```python
from build123d import *

# Parameters (mm, degrees)
BOSS_EXTRUDE1_DEPTH                = 12
SKETCH2_R                          = 6
BOSS_EXTRUDE2_DEPTH                = 3
F_6_0_6_DIAMETER_HOLE2_D           = 6
F_6_0_6_DIAMETER_HOLE2_CSINK_D     = 6.05
F_6_0_6_DIAMETER_HOLE2_CSINK_ANGLE = 90
SKETCH7_R                          = 14
SKETCH7_R_2                        = 9
BOSS_EXTRUDE4_DEPTH                = 17.5
BOSS_EXTRUDE6_DEPTH                = 5
SKETCH9_R                          = 9
CUT_EXTRUDE1_DEPTH                 = 30
BOSS_EXTRUDE7_REACH                = 69.941
SKETCH10_W                         = 30
SKETCH10_H                         = 8
FILLET1_R                          = 10


with BuildPart() as part:
    # Sketch1 → Boss-Extrude1 (new body)
    with BuildSketch(Plane(origin=(0, 0, 0), x_dir=(1, 0, 0), z_dir=(0, 1, 0))):
        with BuildLine():
            Line((-34, 30), (34, 30))
            ThreePointArc((34, 30), (38.242640687, 28.242640687), (40, 24))
            Line((40, 24), (40, -24))
            ThreePointArc((40, -24), (38.242640687, -28.242640687), (34, -30))
            Line((34, -30), (-34, -30))
            ThreePointArc((-34, -30), (-38.242640687, -28.242640687), (-40, -24))
            Line((-40, -24), (-40, 24))
            ThreePointArc((-40, 24), (-38.242640687, 28.242640687), (-34, 30))
        make_face()
    extrude(amount=BOSS_EXTRUDE1_DEPTH)

    # Sketch2 → Boss-Extrude2 (add)
    with BuildSketch(Plane(origin=(0, 12, 0), x_dir=(1, 0, 0), z_dir=(0, 1, 0))):
        with Locations(Location((-34, 24, 0), (0, 0, 90))):
            Circle(SKETCH2_R)
        with Locations(Location((-34, -24, 0), (0, 0, 270))):
            Circle(SKETCH2_R)
        with Locations(Location((34, 24, 0), (0, 0, 90))):
            Circle(SKETCH2_R)
        with Locations(Location((34, -24, 0), (0, 0, 270))):
            Circle(SKETCH2_R)
    extrude(amount=BOSS_EXTRUDE2_DEPTH)

    # Ø6.0 (6) Diameter Hole2 (through all)
    with Locations(Plane(origin=(0, 15, 0), x_dir=(1, 0, 0), z_dir=(0, 1, 0))):
        with Locations((-34, 24), (34, 24), (34, -24), (-34, -24)):
            CounterSinkHole(F_6_0_6_DIAMETER_HOLE2_D / 2, F_6_0_6_DIAMETER_HOLE2_CSINK_D / 2, counter_sink_angle=F_6_0_6_DIAMETER_HOLE2_CSINK_ANGLE)


with BuildPart() as body_2:
    # Sketch7 → Boss-Extrude4 (new, symmetric)
    with BuildSketch(Plane(origin=(0, 0, 0), x_dir=(0, 0, -1), z_dir=(1, 0, 0))):
        with Locations((0, 40)):
            Circle(SKETCH7_R)
        with Locations((0, 40)):
            Circle(SKETCH7_R_2, mode=Mode.SUBTRACT)
    extrude(amount=BOSS_EXTRUDE4_DEPTH, both=True)

    # Sketch8 → Boss-Extrude6 (add, symmetric)
    with BuildSketch(Plane(origin=(0, 0, 0), x_dir=(0, 0, -1), z_dir=(1, 0, 0))):
        with BuildLine():
            Line((-18, 40), (-18, 58))
            Line((-18, 58), (18, 58))
            Line((18, 58), (18, 40))
            ThreePointArc((18, 40), (0, 22), (-18, 40))
        make_face()
    extrude(amount=BOSS_EXTRUDE6_DEPTH, both=True)

    # Sketch9 → Cut-Extrude1 (cut, symmetric)
    with BuildSketch(Plane(origin=(5, 0, 0), x_dir=(0, 0, -1), z_dir=(1, 0, 0))):
        with Locations((0, 40)):
            Circle(SKETCH9_R)
    extrude(amount=CUT_EXTRUDE1_DEPTH, both=True, mode=Mode.SUBTRACT)

    # Sketch10 → Boss-Extrude7 (add, up to next)
    with BuildSketch(Plane(origin=(0, 12, 0), x_dir=(1, 0, 0), z_dir=(0, 1, 0)), mode=Mode.PRIVATE) as boss_extrude7_sk1:
        Rectangle(SKETCH10_W, SKETCH10_H)
    boss_extrude7_tool1 = extrude(boss_extrude7_sk1.sketch, amount=BOSS_EXTRUDE7_REACH, mode=Mode.PRIVATE) - body_2.part

    add(part.part)  # Boss-Extrude7 merges part
    add(boss_extrude7_tool1.solids().sort_by_distance((0, 12, 0))[0])

    # Fillet1
    fillet1_edges = [body_2.edges().sort_by_distance(p)[0] for p in [
        (0, 58, 18),
        (0, 58, -18),
    ]]
    fillet(fillet1_edges, radius=FILLET1_R)


solid = body_2.part
```
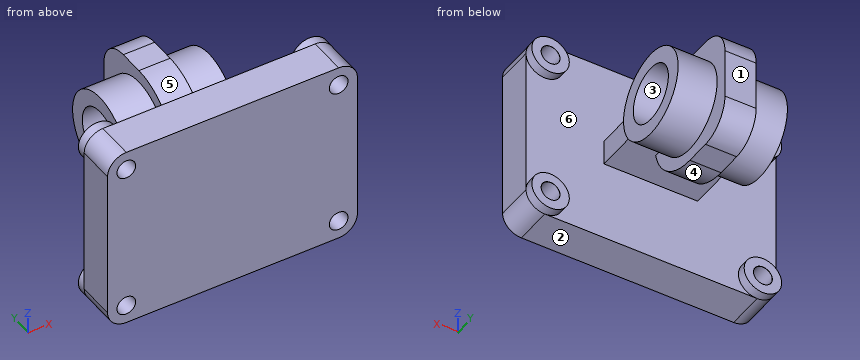
Check sheet for the modelled part. Datum: model origin and axes. Units: mm. Face numbers are marked on the shaded views. A direction names the side the tool comes from. Coordinates: 2 decimals unless noted, no trailing zeros. Order: outer loops, then holes, each group sorted by start corner. A loop starts at its lowest first (then second) coordinate and runs counter-clockwise, first axis right, second up. Notation, with made-up numbers: M 68,38.5 L 83,38.5 A9 cw 83,46.5 Z; hole C 35.25,64 d9. An arc over 180 degrees is marked long. Write each question's results on one line, items separated by ' | '. Start each with the question number.
1. Cross-section at B-B on x = 14. Record the cut outline in (y, z), and give its area (3 significant figures).
2. Access from +Z, -Z, +X, -X, +Y, -Y to the whole of each face (thin tool, end or side, straight path). Record for the marked faces 4, 5 and 6.
3. Cross-section at A-A on z = 0. Record the cut outline in (x, y).
4. Cross-section at D-D on y = 32.5. Record the cut outline in (x, z), and give its area (3 significant figures).
5. Mould release check, pull along Y, two halves, no side actions. Record for the marked faces 1, 2 and 3: +Y half, -Y half, draft (parallel to the pull), parting line (faces both ways), or undercut.
6. Cross-section at C-C on y = 9. Record the cut outline in (x, z).
7. Go/stop test with flat-tipped pins: P1, Ø18, axis at y = 32, z = -4.5, coming from the +X side; P2, Ø3.5, axis at x = -34, z = -24, coming from the +Y side; P3, Ø6, axis at x = 33.5, z = 22, coming from the +Y side; P4, Ø3, axis at x = 21.5, z = -9.5, coming from the +Y side. Record where each tip stops, or that it passes through.
8. Material ranges on probe 1 along Z at (x, y) = (34, 10); probe 2 along X at (y, z) = (4.75, -24); probe 3 along Y at (x, z) = (3, 0), recorded low to high.
Checks:
1) outline: M 0,-30 L 12,-30 L 12,-4 L 26.58,-4 A14 ccw long 26.58,4 L 12,4 L 12,30 L 0,30 Z; hole C 40,0 d18 | area: 1,190 mm²
2) face 4: -Z, +X, -X | face 5: +Z, +X, -X | face 6: none
3) outline: M -40,0 L 40,0 L 40,12 L 15,12 L 15,26 L 17.5,26 L 17.5,31 L -17.5,31 L -17.5,26 L -15,26 L -15,12 L -40,12 Z; M -17.5,49 L 17.5,49 L 17.5,54 L 5,54 L 5,58 L -5,58 L -5,54 L -17.5,54 Z
4) outline: M -17.5,-11.82 L -5,-11.82 L -5,-16.36 L 5,-16.36 L 5,-11.82 L 17.5,-11.82 L 17.5,-4.97 L -17.5,-4.97 Z; M -17.5,4.97 L 17.5,4.97 L 17.5,11.82 L 5,11.82 L 5,16.36 L -5,16.36 L -5,11.82 L -17.5,11.82 Z | area: 570 mm²
5) face 1: +Y half | face 2: draft | face 3: undercut
6) outline: M -40,-24 A6 ccw -34,-30 L 34,-30 A6 ccw 40,-24 L 40,24 A6 ccw 34,30 L -34,30 A6 ccw -40,24 Z; hole C -34,-24 d6; hole C -34,24 d6; hole C 34,-24 d6; hole C 34,24 d6
7) P1: stops at x = 17.5 | P2: passes through | P3: stops at y = 15 | P4: stops at y = 12
8) probe 1: z = -30 to -27, -21 to 21, 27 to 30 | probe 2: x = -40 to -37, -31 to 31, 37 to 40 | probe 3: y = 0 to 31, 49 to 58
